from build123d import *

# Parameters (mm, degrees)
SKETCH2_R             = 3
BOSS_EXTRUDE1_DEPTH   = 25
SKETCH5_W             = 200
SKETCH5_H             = 50
CUT_EXTRUDE1_DEPTH    = 8
SKETCH9_W             = 20.5
SKETCH9_H             = 26.5
BATTERY_DEPTH         = 4.5
SKETCH8_W             = 15.5
SKETCH8_H             = 15.5
TEG_TOP_MIDDLE_DEPTH  = 4.5
SKETCH10_W            = 20.5
SKETCH10_H            = 30.5
POWPCB_NEXTBATT_DEPTH = 4.5
SKETCH12_W            = 247.875067181
SKETCH12_H            = 102.432022038
CUT_EXTRUDE2_DEPTH    = 14
SKETCH13_W            = 7.9930444
SKETCH13_H            = 8
SKETCH13_W_2          = 5.289616262
BOSS_EXTRUDE2_DEPTH   = 51
SKETCH14_W            = 3.79
SKETCH14_H            = 8.67
BOSS_EXTRUDE3_DEPTH   = 8
SKETCH15_W            = 3.67
SKETCH15_H            = 8.67
BOSS_EXTRUDE4_DEPTH   = 9


with BuildPart() as part:
    # Sketch2 → Boss-Extrude1 (new body)
    with BuildSketch(Plane(origin=(0, 0, 0), x_dir=(1, 0, 0), z_dir=(0, 1, 0))):
        with BuildLine():
            Line((-31.5, -35), (31.5, -35))
            ThreePointArc((31.5, -35), (35.035533906, -33.535533906), (36.5, -30))
            Line((36.5, -30), (36.5, 30))
            ThreePointArc((36.5, 30), (35.035533906, 33.535533906), (31.5, 35))
            Line((31.5, 35), (-31.5, 35))
            ThreePointArc((-31.5, 35), (-35.035533906, 33.535533906), (-36.5, 30))
            Line((-36.5, 30), (-36.5, -30))
            ThreePointArc((-36.5, -30), (-35.035533906, -33.535533906), (-31.5, -35))
        make_face()
        with Locations((-31.5, 30)):
            Circle(SKETCH2_R, mode=Mode.SUBTRACT)
        with Locations((-31.5, -30)):
            Circle(SKETCH2_R, mode=Mode.SUBTRACT)
        with Locations((31.5, 30)):
            Circle(SKETCH2_R, mode=Mode.SUBTRACT)
        with Locations((31.5, -30)):
            Circle(SKETCH2_R, mode=Mode.SUBTRACT)
    extrude(amount=BOSS_EXTRUDE1_DEPTH)

    # Sketch5 → Cut-Extrude1 (cut)
    with BuildSketch(Plane(origin=(0, 25, 0), x_dir=(1, 0, 0), z_dir=(0, 1, 0))):
        Rectangle(SKETCH5_W, SKETCH5_H)
    extrude(amount=-CUT_EXTRUDE1_DEPTH, mode=Mode.SUBTRACT)

    # Sketch9 → Battery (add)
    with BuildSketch(Plane(origin=(78.136647367, 17, 0), x_dir=(1, 0, 0), z_dir=(0, 1, 0))):
        with Locations((-65.5549825, -9.238518767)):
            Rectangle(SKETCH9_W, SKETCH9_H)
    extrude(amount=BATTERY_DEPTH)

    # Sketch8 → TEG(Top Middle) (add)
    with BuildSketch(Plane(origin=(0.095109107, 17, -16.130780733), x_dir=(1, 0, 0), z_dir=(0, 1, 0))):
        with Locations((12.905058884, -1.308244326)):
            Rectangle(SKETCH8_W, SKETCH8_H)
    extrude(amount=TEG_TOP_MIDDLE_DEPTH)

    # Sketch10 → PowPCB(nextbatt) (add)
    with BuildSketch(Plane(origin=(-57.874767331, 17, 5.938113267), x_dir=(1, 0, 0), z_dir=(0, 1, 0))):
        with Locations((48.479710494, 5)):
            Rectangle(SKETCH10_W, SKETCH10_H)
    extrude(amount=POWPCB_NEXTBATT_DEPTH)

    # Sketch12 → Cut-Extrude2 (cut)
    with BuildSketch(Plane.XZ):
        with Locations((-0.926975658, -6.36803857)):
            Rectangle(SKETCH12_W, SKETCH12_H)
    extrude(amount=-CUT_EXTRUDE2_DEPTH, mode=Mode.SUBTRACT)

    # Sketch13 → Boss-Extrude2 (add)
    with BuildSketch(Plane(origin=(0, 0, 25), x_dir=(-1, 0, 0), z_dir=(0, 0, -1))):
        with Locations((32.5034778, 21)):
            Rectangle(SKETCH13_W, SKETCH13_H)
        with Locations((-33.855191869, 21)):
            Rectangle(SKETCH13_W_2, SKETCH13_H)
    extrude(amount=BOSS_EXTRUDE2_DEPTH)

    # Sketch14 → Boss-Extrude3 (add)
    with BuildSketch(Plane(origin=(0, 17, 0), x_dir=(1, 0, 0), z_dir=(0, 1, 0))):
        with Locations((-24.424089145, -13.560130433)):
            Rectangle(SKETCH14_W, SKETCH14_H)
        with Locations((-24.424089145, 11.779869567)):
            Rectangle(SKETCH14_W, SKETCH14_H)
        with Locations((-24.424089145, -0.890130433)):
            Rectangle(SKETCH14_W, SKETCH14_H)
    extrude(amount=BOSS_EXTRUDE3_DEPTH)

    # Sketch15 → Boss-Extrude4 (add)
    with BuildSketch(Plane(origin=(49.484284455, 25, 12.830577775), x_dir=(1, 0, 0), z_dir=(0, 1, 0))):
        with Locations((-22.856133, 0.894138312)):
            Rectangle(SKETCH15_W, SKETCH15_H)
        with Locations((-22.856133, 26.234138312)):
            Rectangle(SKETCH15_W, SKETCH15_H)
        with Locations((-22.856133, 13.564138312)):
            Rectangle(SKETCH15_W, SKETCH15_H)
    extrude(amount=-BOSS_EXTRUDE4_DEPTH)


solid = part.part
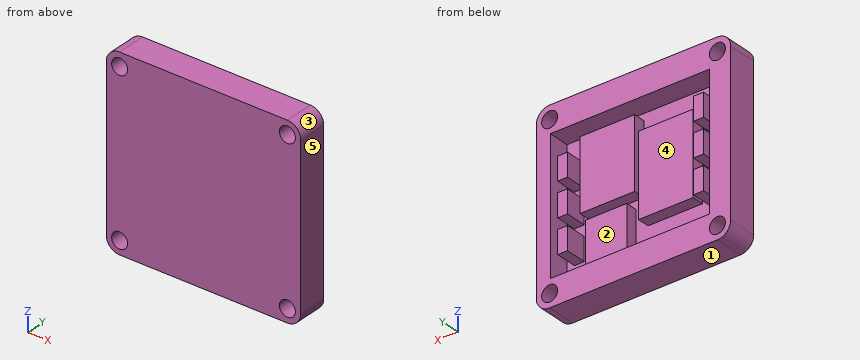
The listing builds one solid part. Answer for the finished solid, in the listing's coordinates (mm). Face numbers are marked on the shaded views. A direction names the side the tool comes from. Round coordinates to 2 decimals unless told otherwise and drop trailing zeros. Write each loop counter-clockwise with the first axis right and the second up, starting at its lowest first coordinate (ties: lowest second). Pieces come first, ordered by that corner, then holes. Notation, with made-up numbers: M -1.5,14 L 23.5,14 A23 ccw 23.5,22 Z; hole C 26,20 d6. An arc over 180 degrees is marked long. Write each question's results on one line, items separated by ' | '. Start each with the question number.
Item 1: Flat-ended cylindrical pins translate along their axes: pin 1 Ø12.5 at (x, z) = (9.5, -17.5) entering from +Y; pin 2 Ø5.5 at (x, z) = (31.5, 30) entering from -Y. Find the tip coordinate at first contact, or state that the pin passes through.
Item 2: A cutting plane is placed at A-A on y = 15.75. Write down the section's boundary in (x, z), and give its area (3 significant figures).
Item 3: A cutting plane is placed at B-B on z = -21.5. Write down the section's boundary in (x, y).
Item 4: A cutting plane is placed at C-C on x = -27.5. Write down the section's boundary in (y, z).
Item 5: For a pull along Z with two mould halves and no side action, classify the marked faces 3, 4 and 5 as pulls with the +Z half, pulls with the -Z half, needs draft (parallel to the pull), parting line crosses it, or undercut.
Item 6: Straight lines are drawn through the part: L1, parallel to X at y = 20.5, z = 4; L2, parallel to Z at x = 31.5, y = 18.5; L3, parallel to X at y = 22, z = 16. For each, find the intervals that lie inside material, in ascending order. Write a range as [from, to].
Item 7: For the marked faces 1 and 2, determine the directions among +Z, -Z, +X, -X, +Y, -Y from which every point of the face is accessible in a straight line to the end or side of a thin tool.
Item 8: A cutting plane is placed at D-D on z = 1. Write down the section's boundary in (x, y).
Check sheet entries:
1) pin 1: y = 21.5 | pin 2: through
2) outline: M -36.5,-30 A5 ccw -31.5,-35 L 31.5,-35 A5 ccw 36.5,-30 L 36.5,30 A5 ccw 31.5,35 L -31.5,35 A5 ccw -36.5,30 Z; hole C -31.5,-30 d6; hole C -31.5,30 d6; hole C 31.5,-30 d6; hole C 31.5,30 d6 | area: 4,980 mm²
3) outline: M -36.5,14 L 36.5,14 L 36.5,25 L 31.21,25 L 31.21,17 L 20.75,17 L 20.75,21.5 L 5.25,21.5 L 5.25,17 L -28.51,17 L -28.51,25 L -36.5,25 Z
4) outline: M 14,-35 L 25,-35 L 25,-25 L 17,-25 L 17,25 L 25,25 L 25,35 L 14,35 Z
5) face 3: pulls with the +Z half | face 4: undercut | face 5: needs draft
6) L1: [-36.5, -28.51], [-26.32, -22.53], [-19.65, 0.85], [2.33, 22.83], [31.21, 36.5] | L2: [-35, -33], [-27, 27], [33, 35] | L3: [-36.5, -28.51], [-26.32, -22.53], [24.79, 28.46], [31.21, 36.5]
7) face 1: -Z, +X, -X, +Y, -Y | face 2: +Y
8) outline: M -36.5,14 L 36.5,14 L 36.5,25 L 31.21,25 L 31.21,17 L 28.46,17 L 28.46,25 L 24.79,25 L 24.79,17 L 22.83,17 L 22.83,21.5 L 2.33,21.5 L 2.33,17 L 0.85,17 L 0.85,21.5 L -19.65,21.5 L -19.65,17 L -22.53,17 L -22.53,25 L -26.32,25 L -26.32,17 L -28.51,17 L -28.51,25 L -36.5,25 Z
